```python
from build123d import *

# Parameters (mm, degrees)
SKETCH_W        = 120.65
SKETCH_H        = 50.8
PAD_DEPTH       = 20.32
POCKET_DEPTH    = 11.684
SKETCH002_R     = 13.97
POCKET001_DEPTH = 50.801
SKETCH003_R     = 3.175
SKETCH003_R_2   = 5
POCKET002_DEPTH = 20.321
SKETCH004_R     = 6.25
POCKET003_DEPTH = 3.556
CHAMFER_SIZE    = 3.048


with BuildPart() as part:
    # Sketch → Pad (new body)
    with BuildSketch(Plane.XY):
        Rectangle(SKETCH_W, SKETCH_H)
    extrude(amount=PAD_DEPTH)

    # Sketch001 (on Face6 of Pad) → Pocket (cut)
    with BuildSketch(Plane.XY.offset(20.32)):
        with BuildLine():
            Line((21.59, -11.43), (21.59, -25.4))
            Line((21.59, -25.4), (-21.59, -25.4))
            Line((-21.59, -25.4), (-21.59, -11.43))
            ThreePointArc((21.59, -11.43), (0, 10.16), (-21.59, -11.43))
        make_face()
    extrude(amount=-POCKET_DEPTH, mode=Mode.SUBTRACT)

    # Sketch002 (on Face6 of Pocket) → Pocket001 (cut, through all)
    with BuildSketch(Plane.XZ.offset(25.4)):
        with Locations((48.5013, 20.32)):
            Circle(SKETCH002_R)
        with Locations((-48.5013, 20.32)):
            Circle(SKETCH002_R)
    extrude(amount=-POCKET001_DEPTH, mode=Mode.SUBTRACT)

    # Sketch003 (on Face5 of Pocket001) → Pocket002 (cut, through all)
    with BuildSketch(Plane.XY.offset(20.32)):
        with Locations((-29.972, 17.78)):
            Circle(SKETCH003_R)
        with Locations((0, 17.78)):
            Circle(SKETCH003_R)
        with Locations((29.972, 17.78)):
            Circle(SKETCH003_R)
        with Locations((-29.972, -11.43)):
            Circle(SKETCH003_R)
        with Locations((0, -11.43)):
            Circle(SKETCH003_R_2)
        with Locations((29.972, -11.43)):
            Circle(SKETCH003_R)
    extrude(amount=-POCKET002_DEPTH, mode=Mode.SUBTRACT)

    # Sketch004 (on Face2 of Pocket002) → Pocket003 (cut)
    with BuildSketch(Plane(origin=(0, 0, 0), x_dir=(1, 0, 0), z_dir=(0, 0, -1))):
        with Locations((0, 11.43)):
            Circle(SKETCH004_R)
    extrude(amount=-POCKET003_DEPTH, mode=Mode.SUBTRACT)

    # Chamfer
    chamfer_edges = [part.edges().sort_by_distance(p)[0] for p in [
        (-5, -11.43, 8.636),
    ]]
    chamfer(chamfer_edges, length=CHAMFER_SIZE)


solid = part.part
```
Can you work these out from the model? Positions are in its coordinate system, mm. A direction names the side the tool comes from. Give positions to 0.01 mm unless a question says otherwise; leave off trailing zeros. Loops run counter-clockwise (first coordinate to the right, second up) from the corner with the lowest first, then second, coordinate; pieces in that order, holes last. Notation, with made-up numbers: M 3.25,13.5 L 19.25,13.5 A13 ccw 19.25,32.5 Z; hole C 9.25,-1.5 d11. An arc over 180 degrees is marked long. One line per question, with ' | ' between items. Start each with the question number.
Q1. If we mould it in two halves opening along Y, with no side actions, what happens to faces 4 (the flat face through (-4, -3, 8.636)), 5 (the cylindrical face through (-1.08, -16.31, 4.59)), 6 (the flat face through (-1, 25.4, 8))? For each: +Y half, -Y half, draft (parallel to the pull), parting line (faces both ways), or undercut.
Q2. If we section it at B-B (y = 17.78): Please give me the cut outline in (x, z) (1 decimal).
Q3. For pin 1 Ø13 at (x, y) = (0, -11.43) entering from +Z; pin 2 Ø8 at (x, y) = (-45.5, 5.5) entering from +Z; pin 3 Ø18 at (x, y) = (10.5, -8) entering from +Z, each with a flat end and sliding along its axis, tell me the tip position at first contact or that it passes through.
Q4. If I drill on line 1 (Y direction, x = 0, z = 2.4) (3 decimals); line 2 (Y direction, x = 0, z = 11) (3 decimals); line 3 (X direction, y = -9.5, z = 12.5) (1 decimal), over which ranges is the centre line in solid material (lowest first)? Write a range as from..to.
Q5. If we section it at D-D (x = 29.5): Please give me the cut outline in (y, z), plus the area to 3 significant figures.
Q6. If we section it at C-C (z = 15.5): Please give me the cut outline in (x, y) (3 decimals).
Q7. If we section it at A-A (x = 0): Please give me the cut outline in (y, z) (3 decimals).
Q8. For faces 1 (the flat face through (21.59, -18, 15)), 2 (the cylindrical face through (-44.87, -0.36, 6.83)), 3 (the flat face through (-3, -16, 3.556)), which set-ups out of +Z, -Z, +X, -X, +Y, -Y let a thin tool reach every point of the face, with its end or its side?
Computed:
1) face 4: draft | face 5: undercut | face 6: +Y half
2) outline: M -60.3,0 L -33.1,0 L -33.1,20.3 L -34.5,20.3 A14 cw -60.3,12.9 Z; M -26.8,0 L -3.2,0 L -3.2,20.3 L -26.8,20.3 Z; M 3.2,0 L 26.8,0 L 26.8,20.3 L 3.2,20.3 Z; M 33.1,0 L 60.3,0 L 60.3,12.9 A14 cw 34.5,20.3 L 33.1,20.3 Z
3) pin 1: stops at z = 7.09 | pin 2: stops at z = 8.23 | pin 3: stops at z = 8.64
4) line 1: y = -25.4..-17.68, -5.18..14.605, 20.955..25.4 | line 2: y = 10.16..14.605, 20.955..25.4 | line 3: x = -60.3..-60.1, -36.9..-32.5, -27.5..-21.5, 21.5..27.5, 32.5..36.9, 60.1..60.3
5) outline: M -25.4,0 L -14.57,0 L -14.57,20.32 L -25.4,20.32 Z; M -8.29,0 L 14.64,0 L 14.64,20.32 L -8.29,20.32 Z; M 20.92,0 L 25.4,0 L 25.4,20.32 L 20.92,20.32 Z | area: 777 mm²
6) outline: M -35.389,-25.4 L -21.59,-25.4 L -21.59,-11.43 A21.59 cw 21.59,-11.43 L 21.59,-25.4 L 35.389,-25.4 L 35.389,25.4 L -35.389,25.4 Z; hole C -29.972,-11.43 d6.35; hole C -29.972,17.78 d6.35; hole C 0,17.78 d6.35; hole C 29.972,-11.43 d6.35; hole C 29.972,17.78 d6.35
7) outline: M -25.4,0 L -17.68,0 L -17.68,3.556 L -16.43,3.556 L -16.43,5.588 L -19.478,8.636 L -25.4,8.636 Z; M -6.43,3.556 L -5.18,3.556 L -5.18,0 L 14.605,0 L 14.605,20.32 L 10.16,20.32 L 10.16,8.636 L -3.382,8.636 L -6.43,5.588 Z; M 20.955,0 L 25.4,0 L 25.4,20.32 L 20.955,20.32 Z
8) face 1: +Z, -Y | face 2: +Z, +Y, -Y | face 3: -Z
